Geometry: see drawing. Coordinates: mm, zero at the bounding-box minimum. Coordinates: 2 decimals unless noted, no trailing zeros. Order: outer loops, then holes, each group sorted by start corner. A loop starts at its lowest first (then second) coordinate and runs counter-clockwise, first axis right, second up. Notation, with made-up numbers: (-22.5, 11) -> (4.5, 11) arc R18 ccw to (4.5, 21) -> close; hole circle Ø10 at (26.5, 0.25). An arc over 180 degrees is marked (long way). Write each question's results on one line, items separated by ' | '.
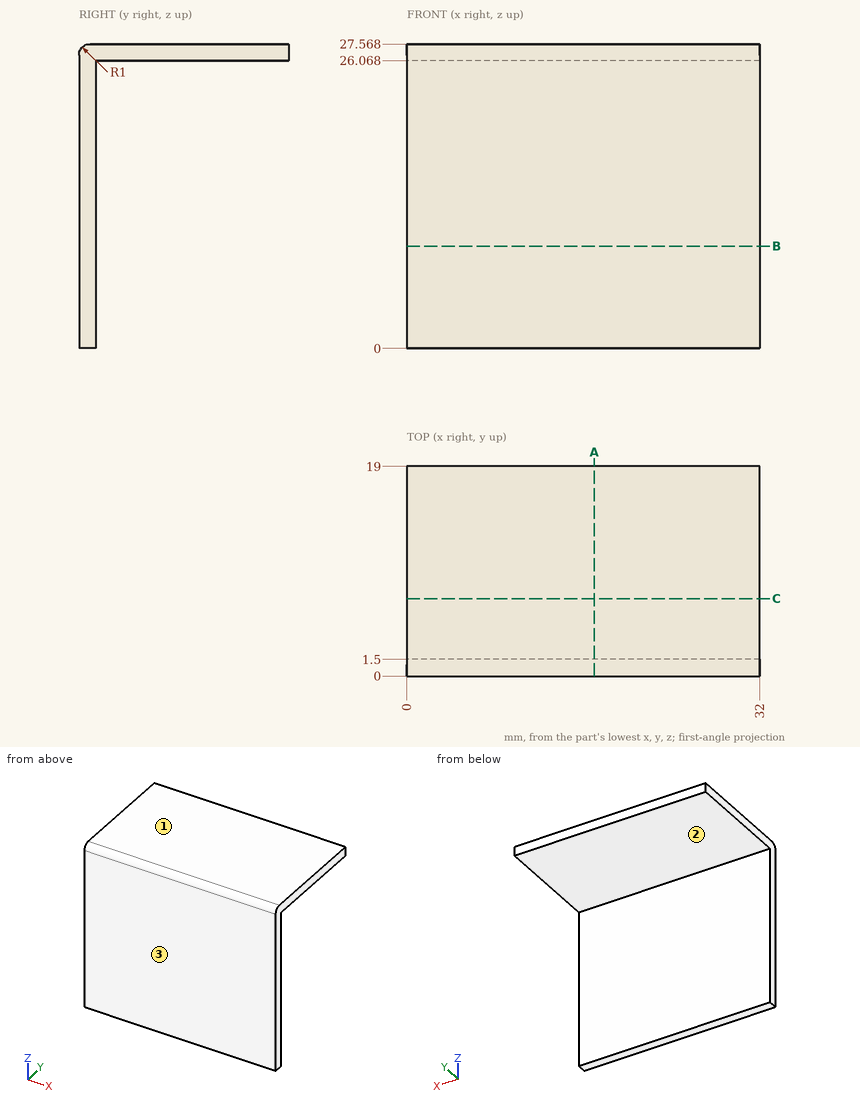
(1) Cut plane B-B, the plane z = 9.25. Return loops of the section in (x, y).
Return value:
outline: (0, 0) -> (32, 0) -> (32, 1.5) -> (0, 1.5) -> close
(2) Line query: line 1 along Z through (x, y) = (30, 3.75); line 2 along Y through (x, z) = (9, 14.5). Output: solid intervals per line, ascending. Write a range as from..to.
Return value:
line 1: 26.07..27.57 | line 2: 0..1.5
(3) Cut plane A-A, the plane x = 17. Return loops of the section in (y, z).
Return value:
outline: (0, 0) -> (1.5, 0) -> (1.5, 26.07) -> (19, 26.07) -> (19, 27.57) -> (1, 27.57) arc R1 ccw to (0, 26.57) -> close
(4) Mould query, pull axis Z, two halves, no side actions, for the marked faces 1, 2 and 3. Classes: +Z half, -Z half, draft (parallel to the pull), parting line (faces both ways), or undercut.
Return value:
face 1: +Z half | face 2: -Z half | face 3: draft
(5) Cut plane C-C, the plane y = 7. Return loops of the section in (x, z).
Return value:
outline: (0, 26.07) -> (32, 26.07) -> (32, 27.57) -> (0, 27.57) -> close
(6) Pin query (flat end, axial travel): P1, Ø1.5, axis at x = 28, z = 10, coming from the +Y side; P2, Ø3, axis at x = 21, z = 16.5, coming from the -Y side. Return the tip coordinate at first contact, or that it passes through.
Return value:
P1: y = 1.5 | P2: y = 0
